For this review, use the dimensioned drawing (mm, ordinates from the lowest corner) and the shaded views. A direction names the side the tool comes from. Coordinates: 2 decimals unless noted, no trailing zeros. Loops run counter-clockwise (first coordinate to the right, second up) from the corner with the lowest first, then second, coordinate; pieces in that order, holes last. Notation, with made-up numbers: (46, 50.5) - (76, 50.5) arc R28 ccw to (76, 71.5) - close; hole circle Ø6 at (69, -9.5). An arc over 180 degrees is marked (long way). Use a Markdown table: item, result. Add a question column.
1) Clearance check with flat-ended pins moving along their axes: pin 1 (8 mm diameter, centred on y = 30, z = 6, fed in from -X); pin 2 (2.5 mm diameter, centred on x = 11, y = 24, fed in from -Z); pin 3 (5 mm diameter, centred on x = 18.5, y = 18.5, fed in from -Z); pin 4 (6 mm diameter, centred on x = 8.5, z = 15.5, fed in from -Y). State where each tip first meets the part, or that it passes through.
2) Add section D-D, the plane x = 15.5. Give the boundary of the cut face in (y, z).
3) To check wall thickness, follow L1, parallel to Y at x = 19.75, z = 3.25; L2, parallel to X at y = 1, z = 20 (1 decimal); L3, parallel to X at y = 31.5, z = 12.25. State the ranges of each line that lie inside material, in increasing order. Write a range as [from, to].
4) For the marked faces 1, 2 and 3, list the 3-axis set-ups (+Z, -Z, +X, -X, +Y, -Y) from which the entire face can be reached by the end or side of a thin tool; tool diameter is ignored.
5) Add section B-B, the plane z = 19.75. Give the boundary of the cut face in (x, y), and give its area (3 significant figures).
6) Add section C-C, the plane z = 13.75. Give the boundary of the cut face in (x, y), and give its area (3 significant figures).
7) Add section A-A, the plane x = 12. Give the boundary of the cut face in (y, z), and give its area (3 significant figures).
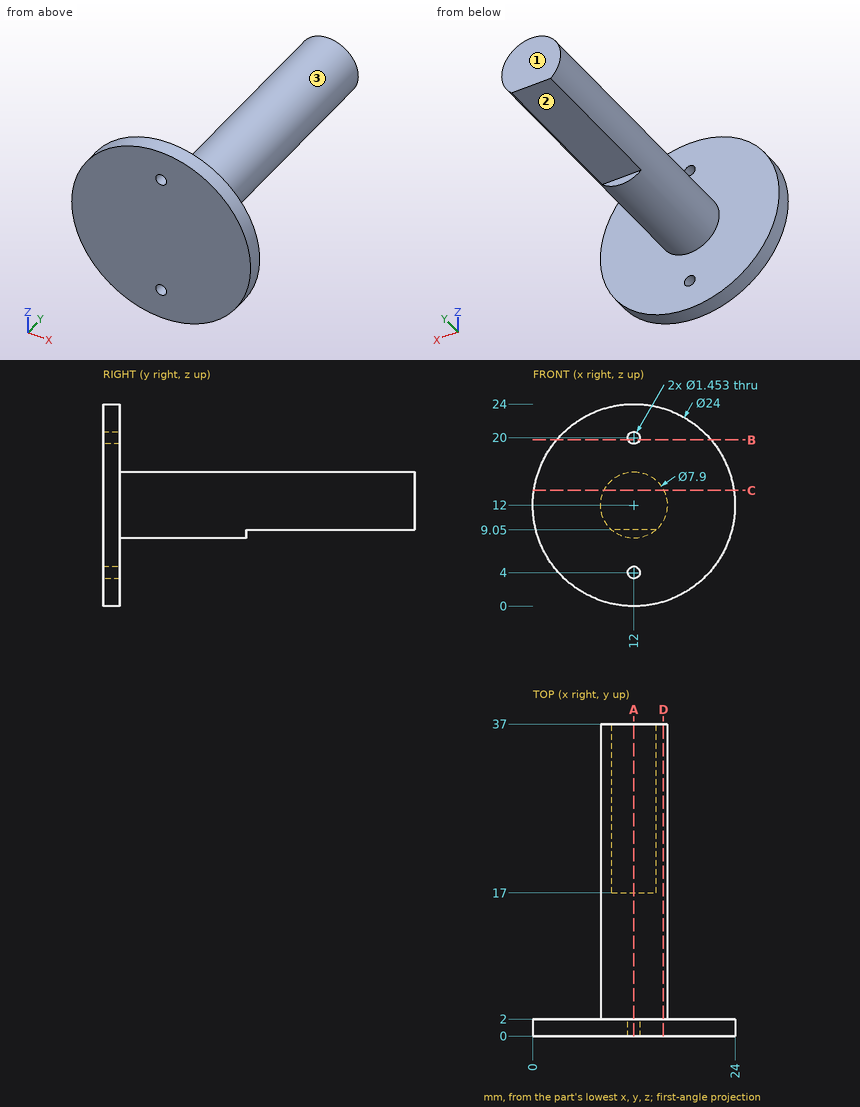
From the geometry:
| question | item | result |
|---|---|---|
| 1 | pin 1 | stops at x = 8.59 |
| 1 | pin 2 | stops at z = 9.05 |
| 1 | pin 3 | passes through |
| 1 | pin 4 | stops at y = 0 |
| 2 | outline | (0, 0.52) - (2, 0.52) - (2, 10.17) - (37, 10.17) - (37, 13.83) - (2, 13.83) - (2, 23.48) - (0, 23.48) - close |
| 3 | L1 | y = [0, 2] |
| 3 | L2 | x = [3.1, 11.3], [12.7, 20.9] |
| 3 | L3 | x = [8.06, 15.94] |
| 4 | face 1 | +Z, -Z, +X, -X, +Y |
| 4 | face 2 | -Z, +X, -X, +Y |
| 4 | face 3 | +Y |
| 5 | outline | (2.84, 0) - (11.32, 0) - (11.32, 2) - (2.84, 2) - close; (12.68, 0) - (21.16, 0) - (21.16, 2) - (12.68, 2) - close |
| 5 | area | 33.9 mm^2 |
| 6 | outline | (0.13, 0) - (23.87, 0) - (23.87, 2) - (15.54, 2) - (15.54, 37) - (8.46, 37) - (8.46, 2) - (0.13, 2) - close |
| 6 | area | 295 mm^2 |
| 7 | outline | (0, 0) - (2, 0) - (2, 3.27) - (0, 3.27) - close; (0, 4.73) - (2, 4.73) - (2, 8.05) - (17, 8.05) - (17, 9.05) - (37, 9.05) - (37, 15.95) - (2, 15.95) - (2, 19.27) - (0, 19.27) - close; (0, 20.73) - (2, 20.73) - (2, 24) - (0, 24) - close |
| 7 | area | 299 mm^2 |
